The listing builds one solid part. Answer for the finished solid, in the listing's coordinates (mm). Coordinates: 2 decimals unless noted, no trailing zeros. Order: outer loops, then holes, each group sorted by start corner. A loop starts at its lowest first (then second) coordinate and runs counter-clockwise, first axis right, second up. Notation, with made-up numbers: (-18.75, 9.25) -> (8.25, 9.25) arc R21 ccw to (8.25, 35.25) -> close; hole circle Ø11 at (84.25, -0.5). An arc over 180 degrees is marked (long way). Write item = value, one per line. Start each with the question number.
```python
from build123d import *

# Parameters (mm, degrees)
EXTRUDE1_DEPTH = 4.5
FILLET1_R      = 0.5


with BuildPart() as part:
    # Sketch2 → Extrude1 (new body)
    with BuildSketch(Plane.XY):
        with BuildLine():
            ThreePointArc((1.467618759, 6.404104167), (0.094372819, 7.528980002), (-0.996737871, 6.128755907))
            ThreePointArc((-0.996737871, 6.128755907), (-0.750709422, -0.125968829), (-1.706502063, -6.312128537))
            ThreePointArc((-1.706502063, -6.312128537), (-1.584231252, -7.071852789), (-0.946059773, -7.501815872))
            ThreePointArc((-0.946059773, -7.501815872), (0.688671474, -7.111598822), (1.495022371, -5.637009447))
            ThreePointArc((1.495022371, -5.637009447), (1.73628539, 0.384127619), (1.467618759, 6.404104167))
        make_face()
    extrude(amount=EXTRUDE1_DEPTH)

    # Fillet1
    fillet1_edges = [part.edges().sort_by_distance(p)[0] for p in [
        (-0.750709422, -0.125968829, 4.5),
        (-1.584231252, -7.071852789, 4.5),
        (0.688671474, -7.111598822, 4.5),
        (1.73628539, 0.384127619, 4.5),
        (0.094372819, 7.528980002, 4.5),
    ]]
    fillet(fillet1_edges, radius=FILLET1_R)


solid = part.part
```
Item 1: For a pull along Y with two mould halves and no side action, classify faces 1 (the cylindrical face through (-0.746, -0.038, 1.972)), 2 (the cylindrical face through (0.669, -7.126, 1.972)), 3 (the cylindrical face through (-1.59, -7.06, 1.97)) as pulls with the +Y half, pulls with the -Y half, needs draft (parallel to the pull), parting line crosses it, or undercut.
Item 2: Section A-A, the plane z = 3.5 is taken. Give the vertices of the cut face in (x, y).
Item 3: Each of these flat-tipped pins is pushed along its axis until it touches: pin 1 (1 mm diameter, centred on x = -1, z = 1.5, fed in from +Y); pin 2 (2 mm diameter, centred on x = 0.5, y = 4.5, fed in from -Z). Where does it stop, or does it pass through?
Item 4: Consider probe 1 along X at (y, z) = (4, 2.55); probe 2 along X at (y, z) = (7, 1.9); probe 3 along Z at (x, y) = (1.4, -5). Determine where each line is inside the solid, lowest interval first.
A:
q1.face_1 = undercut
q1.face_2 = pulls with the -Y half
q1.face_3 = parting line crosses it
q2.outline = (-1.71, -6.31) arc R0.97 ccw to (-0.95, -7.5) arc R2.07 ccw to (1.5, -5.64) arc R71.21 ccw to (1.47, 6.4) arc R1.24 ccw (long way) to (-1, 6.13) arc R32.55 cw to start
q3.pin_1 = 7.3
q3.pin_2 = 0
q4.probe_1 = -0.78 to 1.64
q4.probe_2 = -0.79 to 1.25
q4.probe_3 = 0 to 4.35
